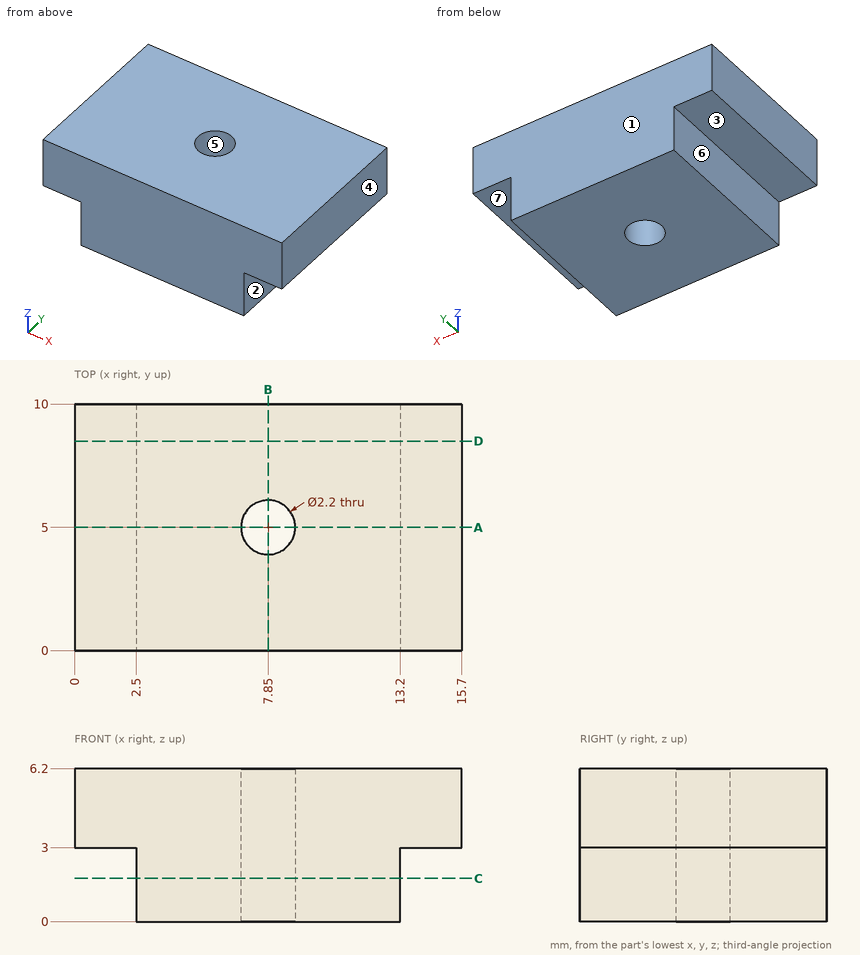
Part print with two shaded views. Sizes in mm from the minimum x, y, z corner. A direction names the side the tool comes from. Coordinates: 2 decimals unless noted, no trailing zeros. Loops run counter-clockwise (first coordinate to the right, second up) from the corner with the lowest first, then second, coordinate; pieces in that order, holes last. Notation, with made-up numbers: M 39.5,-31.75 L 77.5,-31.75 A14 cw 77.5,-4.75 Z; hole C -10.5,27 d10. An arc over 180 degrees is marked long. Use CSV: the item, a comma, the result in double quotes. Start each with the question number.
1. Band-saw the part on C-C, the plane z = 1.75. List the corners of the cut face in (x, y).
2. Band-saw the part on A-A, the plane y = 5. List the corners of the cut face in (x, z).
3. Probe probe 1 along Y at (x, z) = (7.85, 3); probe 2 along Z at (x, y) = (13.5, 8.25); probe 3 along X at (y, z) = (5.5, 0.5). List the from-to ranges inside material, lowest first. Write a range as [from, to].
4. Two-plate mould, pull along X, no slides. Class the marked faces 4, 5, 6 and 7: pulls with the +X half, pulls with the -X half, needs draft (parallel to the pull), parting line crosses it, or undercut.
5. Band-saw the part on B-B, the plane x = 7.85. List the corners of the cut face in (y, z).
6. Tool access for the marked faces 1, 2 and 3: list every direction of +Z, -Z, +X, -X, +Y, -Y with a clear straight run to the whole face (end or side of a thin tool).
7. Flat gauge pins, fed straight in: pin 1 (1 mm diameter, centred on y = 1, z = 2, fed in from +X); pin 2 (1.5 mm diameter, centred on y = 5.5, z = 2, fed in from -X). Where does each tip first touch, or does it go through?
8. Band-saw the part on D-D, the plane y = 8.5. List the corners of the cut face in (x, z).
Entries:
1,outline,"M 2.5,0 L 13.2,0 L 13.2,10 L 2.5,10 Z; hole C 7.85,5 d2.2"
2,outline,"M 0,3 L 2.5,3 L 2.5,0 L 6.75,0 L 6.75,6.2 L 0,6.2 Z; M 8.95,0 L 13.2,0 L 13.2,3 L 15.7,3 L 15.7,6.2 L 8.95,6.2 Z"
3,probe 1,"y = [0, 3.9], [6.1, 10]"
3,probe 2,"z = [3, 6.2]"
3,probe 3,"x = [2.5, 6.87], [8.83, 13.2]"
4,face 4,"pulls with the +X half"
4,face 5,"undercut"
4,face 6,"pulls with the -X half"
4,face 7,"needs draft"
5,outline,"M 0,0 L 3.9,0 L 3.9,6.2 L 0,6.2 Z; M 6.1,0 L 10,0 L 10,6.2 L 6.1,6.2 Z"
6,face 1,"+Z, -Z, +X, -X, +Y"
6,face 2,"-Z, +X, +Y, -Y"
6,face 3,"-Z, -X, +Y, -Y"
7,pin 1,"stops at x = 13.2"
7,pin 2,"stops at x = 2.5"
8,outline,"M 0,3 L 2.5,3 L 2.5,0 L 13.2,0 L 13.2,3 L 15.7,3 L 15.7,6.2 L 0,6.2 Z"
